Geometry: final body of the model. Coordinates: model frame, mm. Face numbers are marked on the shaded views. Coordinates: 2 decimals unless noted, no trailing zeros. Loops run counter-clockwise (first coordinate to the right, second up) from the corner with the lowest first, then second, coordinate; pieces in that order, holes last. Notation, with made-up numbers: (-8, 35.5) -> (20, 35.5) arc R23 ccw to (20, 53.5) -> close; hole circle Ø6 at (-36.5, 8.25). An arc over 180 degrees is marked (long way). One line per item, written item: value. Start each with the question number.
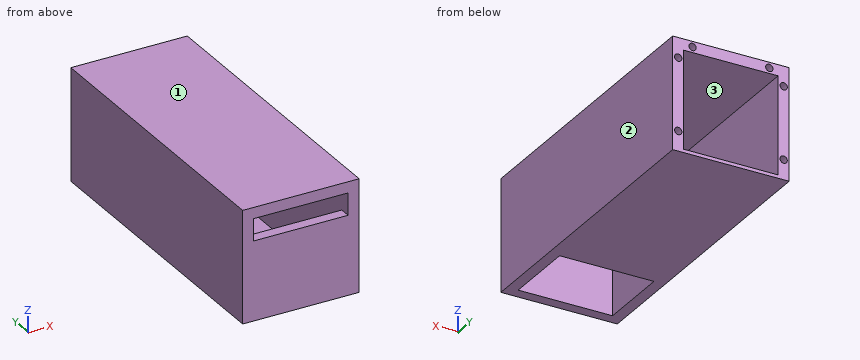
from build123d import *

# Parameters (mm, degrees)
ESQUISSE1_W             = 105.6
ESQUISSE1_H             = 272.4
BOSS_EXTRU_1_DEPTH      = 101.6
ESQUISSE3_W             = 85.6
ESQUISSE3_H             = 88.6
ENL_V_MAT_EXTRU_1_DEPTH = 262.4
ESQUISSE4_W             = 85.6
ESQUISSE4_H             = 20
ENL_V_MAT_EXTRU_2_DEPTH = 30
ESQUISSE5_W             = 85.6
ESQUISSE5_H             = 65.6
ENL_V_MAT_EXTRU_3_DEPTH = 30
D_GAGEMENT_M61_D        = 6.6
D_GAGEMENT_M61_DEPTH    = 10
D_GAGEMENT_M61_TIP      = 1.982840043


with BuildPart() as part:
    # Esquisse1 → Boss.-Extru.1 (new body)
    with BuildSketch(Plane.XY):
        with Locations((-5.189173744, -81.220813953)):
            Rectangle(ESQUISSE1_W, ESQUISSE1_H)
    extrude(amount=BOSS_EXTRU_1_DEPTH)

    # Esquisse3 → Enlèv. mat.-Extru.1 (cut)
    with BuildSketch(Plane(origin=(0, 54.979186047, 0), x_dir=(1, 0, 0), z_dir=(0, 1, 0))):
        with Locations((-5.189173744, -47.3)):
            Rectangle(ESQUISSE3_W, ESQUISSE3_H)
    extrude(amount=-ENL_V_MAT_EXTRU_1_DEPTH, mode=Mode.SUBTRACT)

    # Esquisse4 → Enlèv. mat.-Extru.2 (cut)
    with BuildSketch(Plane.XZ.offset(217.420813953)):
        with Locations((-5.189173744, 81.6)):
            Rectangle(ESQUISSE4_W, ESQUISSE4_H)
    extrude(amount=-ENL_V_MAT_EXTRU_2_DEPTH, mode=Mode.SUBTRACT)

    # Esquisse5 → Enlèv. mat.-Extru.3 (cut)
    with BuildSketch(Plane(origin=(0, 0, 0), x_dir=(-1, 0, 0), z_dir=(0, 0, -1))):
        with Locations((5.189173744, -174.620813953)):
            Rectangle(ESQUISSE5_W, ESQUISSE5_H)
    extrude(amount=-ENL_V_MAT_EXTRU_3_DEPTH, mode=Mode.SUBTRACT)

    # Dégagement M61
    with Locations(Plane(origin=(-52.989173744, 54.979186047, 18), x_dir=(0, 0, 1), z_dir=(0, 1, 0))):
        with Locations((0, 0), (65.6, 0), (0, 95.6), (65.6, 95.6), (78.6, 13), (78.6, 82.6)):
            Hole(D_GAGEMENT_M61_D / 2, depth=D_GAGEMENT_M61_DEPTH)
            with Locations((0, 0, -(D_GAGEMENT_M61_DEPTH + D_GAGEMENT_M61_TIP / 2))):  # 118° drill point
                Cone(0, D_GAGEMENT_M61_D / 2, D_GAGEMENT_M61_TIP, mode=Mode.SUBTRACT)


solid = part.part
1. Line query: L1, parallel to X at y = 49.25, z = 18; L2, parallel to X at y = 52, z = 83; L3, parallel to X at y = -37.5, z = 41.5. Output: solid intervals per line, ascending. Write a range as [from, to].
2. Section D-D on y = -168. Return the cut outline in (x, z).
3. Draft query along Z for the marked faces 1, 2 and 3. Return one class per face: released by +Z, released by -Z, zero draft, split by the parting line, or undercut.
4. Pin query (flat end, axial travel): pin 1 Ø8 at (x, y) = (-42.5, -189.5) entering from -Z; pin 2 Ø5.5 at (x, z) = (29.61, 96.6) entering from +Y; pin 3 Ø4 at (x, z) = (3.5, 58.5) entering from +Y. Return the tip coordinate at first contact, or that it passes through.
5. Section C-C on z = 33.5. Return the cut outline in (x, y).
6. Section B-B on x = 17. Return the cut outline in (y, z).
7. Section A-A on y = -107. Return the cut outline in (x, z).
Checks:
1. L1: [-57.99, -56.29], [-49.69, -47.99], [37.61, 39.31], [45.91, 47.61]
1. L2: [-57.99, -56.23], [-49.74, -47.99], [37.61, 39.37], [45.86, 47.61]
1. L3: [-57.99, -47.99], [37.61, 47.61]
2. outline: (-57.99, 0) -> (-47.99, 0) -> (-47.99, 91.6) -> (37.61, 91.6) -> (37.61, 0) -> (47.61, 0) -> (47.61, 101.6) -> (-57.99, 101.6) -> close
3. face 1: released by +Z
3. face 2: zero draft
3. face 3: undercut
4. pin 1: z = 91.6
4. pin 2: y = 44.65
4. pin 3: y = -207.42
5. outline: (-57.99, -217.42) -> (47.61, -217.42) -> (47.61, 54.98) -> (37.61, 54.98) -> (37.61, -207.42) -> (-47.99, -207.42) -> (-47.99, 54.98) -> (-57.99, 54.98) -> close
6. outline: (-217.42, 0) -> (-207.42, 0) -> (-207.42, 71.6) -> (-217.42, 71.6) -> close; (-217.42, 91.6) -> (54.98, 91.6) -> (54.98, 101.6) -> (-217.42, 101.6) -> close; (-141.82, 0) -> (54.98, 0) -> (54.98, 3) -> (-141.82, 3) -> close
7. outline: (-57.99, 0) -> (47.61, 0) -> (47.61, 101.6) -> (-57.99, 101.6) -> close; hole (-47.99, 3) -> (37.61, 3) -> (37.61, 91.6) -> (-47.99, 91.6) -> close
